from build123d import *

# Parameters (mm, degrees)
SKETCH_2_R      = 2
EXTRUDE_1_DEPTH = 1.5


with BuildPart() as part:
    # 草图1 → 旋转1 (revolve)
    with BuildSketch(Plane.XY):
        with BuildLine():
            Line((0, 0), (-14, 0))
            Line((-14, 0), (-14, 8.666286))
            ThreePointArc((-14, 8.666286), (-11.155416, 12.918811), (-7.071068, 16))
            ThreePointArc((-7.071068, 16), (-4.330127, 19.623724), (0, 21))
            Line((0, 21), (0, 0))
        make_face()
    revolve(axis=Axis((0, 0, 0), (0, 1, 0)))

    # 草图2 → 凸台-拉伸1 (add)
    with BuildSketch(Plane(origin=(0, 0, 0), x_dir=(1, 0, 0), z_dir=(0, 1, 0))):
        with BuildLine():
            Line((3.464435, 21.999422), (11.980808, 7.242943))
            ThreePointArc((11.980808, 7.242943), (14, 0), (11.980808, -7.242943))
            Line((11.980808, -7.242943), (3.464435, -21.999422))
            ThreePointArc((3.464435, -21.999422), (0, -24), (-3.464435, -21.999422))
            Line((-3.464435, -21.999422), (-11.980808, -7.242943))
            ThreePointArc((-11.980808, -7.242943), (-14, 0), (-11.980808, 7.242943))
            Line((-11.980808, 7.242943), (-3.464435, 21.999422))
            ThreePointArc((-3.464435, 21.999422), (0, 24), (3.464435, 21.999422))
        make_face()
        with Locations((0, 20)):
            Circle(SKETCH_2_R, mode=Mode.SUBTRACT)
        with Locations((0, -20)):
            Circle(SKETCH_2_R, mode=Mode.SUBTRACT)
    extrude(amount=EXTRUDE_1_DEPTH)


solid = part.part
Here's how the part is built. I have some questions about the finished solid (model axes, mm). A direction names the side the tool comes from. Round coordinates to 2 decimals unless told otherwise and drop trailing zeros. Order: outer loops, then holes, each group sorted by start corner. A loop starts at its lowest first (then second) coordinate and runs counter-clockwise, first axis right, second up. Notation, with made-up numbers: M -3,17.5 L 2,17.5 A23 cw 2,36.5 Z; hole C 59.25,-3 d3. An arc over 180 degrees is marked long. Return JSON: item names as keys, results as strings. Group by question number.
1. I'm going to push flat-ended pins straight in: pin 1 Ø12 at (x, z) = (-4, 11.5) entering from +Y; pin 2 Ø8 at (x, z) = (-5, 10.5) entering from +Y; pin 3 Ø3 at (x, z) = (0, 20) entering from -Y; pin 4 Ø10 at (y, z) = (6, -10) entering from +X. Where does each tip first touch, or does it pass through?
2. On a 3-axis mill with a long thin cutter (end or side, diameter ignored), from which of +Z, -Z, +X, -X, +Y, -Y can I reach the whole of each face in a straight line? I mean faces 1 (the face through (-12.932, 4.394, -5.362)), 2 (the face through (-7.663, 0.74, 14.724)). Say none if no direction works.
3. Please list where these lines run through material, in increasing order: probe 1 along Y at (x, z) = (-3.25, -19.5); probe 2 along Z at (x, y) = (-9.75, 11.75); probe 3 along X at (y, z) = (0.65, 20).
4. If we mould it in two halves opening along X, with no side actions, what happens to faces 3 (the face through (0, 1, -24)), 4 (the face through (7.78, 0.74, 14.52)), 5 (the face through (0, 1.5, -17)), 6 (the face through (0, 1, -22))? For each: pulls with the +X half, pulls with the -X half, needs draft (parallel to the pull), parting line crosses it, or undercut.
5. If we section it at C-C on z = -14.5: List the corners of the cut face in (x, y) for me.
6. If we section it at A-A on z = -20: List the corners of the cut face in (x, y) for me.
7. If we section it at B-B on y = 3.25: List the corners of the cut face in (x, z) for me.
Reply:
{
 "1": {"pin 1": "y = 17.76", "pin 2": "y = 15.7", "pin 3": "through", "pin 4": "x = 13.08"},
 "2": {"face 1": "+Y", "face 2": "+Z, -X, +Y, -Y"},
 "3": {"probe 1": "0 to 1.5", "probe 2": "-7.26 to 7.26", "probe 3": "-4.62 to -2, 2 to 4.62"},
 "4": {"face 3": "parting line crosses it", "face 4": "pulls with the +X half", "face 5": "needs draft", "face 6": "undercut"},
 "5": {"outline": "M -7.79,0 L 7.79,0 L 7.79,1.5 L -7.79,1.5 Z"},
 "6": {"outline": "M -4.62,0 L -2,0 L -2,1.5 L -4.62,1.5 Z; M 2,0 L 4.62,0 L 4.62,1.5 L 2,1.5 Z"},
 "7": {"outline": "C 0,0 d28"}
}
